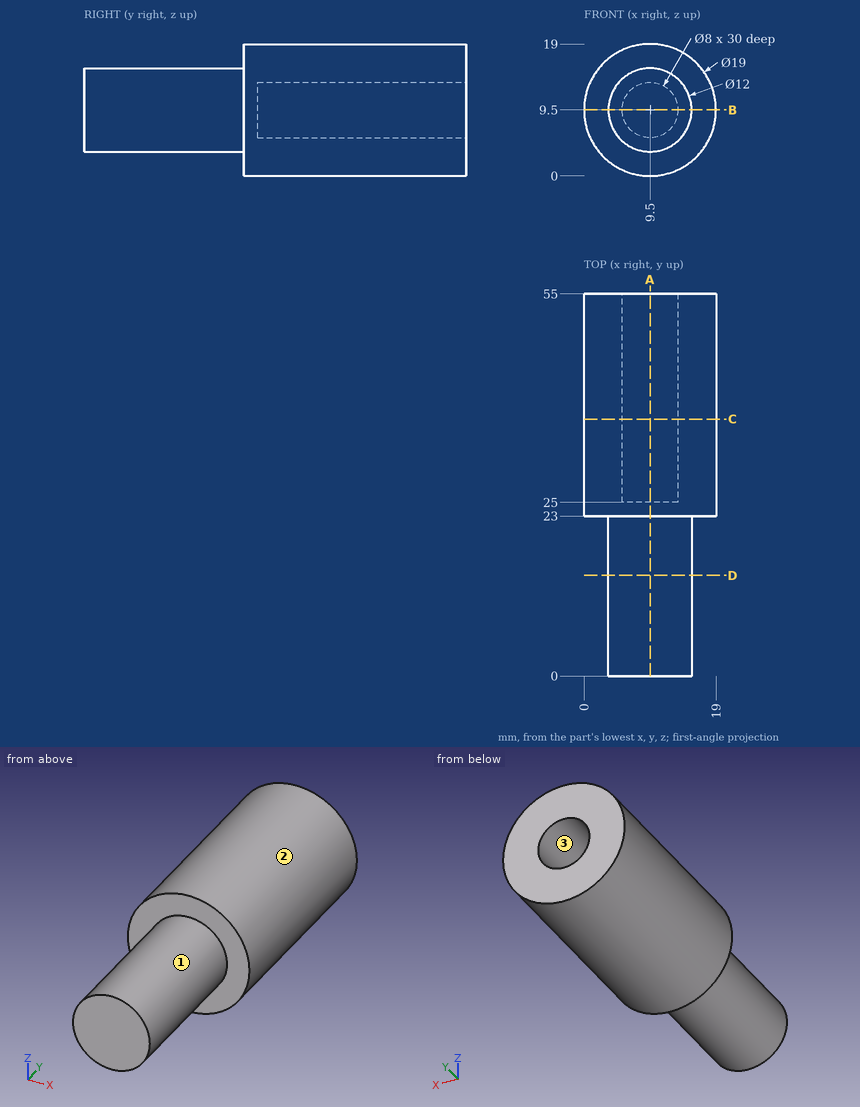
Could you check a few things on this drawing? It's one solid part, dimensions in mm from its lowest x, y, z. A direction names the side the tool comes from. Round coordinates to 2 decimals unless told otherwise and drop trailing zeros. Loops run counter-clockwise (first coordinate to the right, second up) from the corner with the lowest first, then second, coordinate; pieces in that order, holes last. Notation, with made-up numbers: M 43.5,28.5 L 79.5,28.5 A16 ccw 79.5,34.5 Z; hole C 40,35 d4. An arc over 180 degrees is marked long. Write each question's results on one line, items separated by ' | '. Start each with the question number.
(1) Will these pins go through, and if not, where does the flat tip stop? P1, Ø3, axis at y = 25.5, z = 4, coming from the -X side; P2, Ø5, axis at y = 35, z = 13.5, coming from the +X side; P3, Ø3, axis at y = 16, z = 3.5, coming from the -X side.
(2) On a 3-axis mill with a long thin cutter (end or side, diameter ignored), from which of +Z, -Z, +X, -X, +Y, -Y can I reach the whole of each face in a straight line? I mean the marked faces 1, 2 and 3. Say none if no direction works.
(3) I want a section at A-A (x = 9.5). Please give me the cut outline in (y, z), then the cut area to 3 significant figures.
(4) I want a section at D-D (y = 14.5). Please give me the cut outline in (x, z).
(5) I want a section at B-B (z = 9.5). Please give me the cut outline in (x, y), then the cut area to 3 significant figures.
(6) I want a section at C-C (y = 37). Please give me the cut outline in (x, z), then the cut area to 3 significant figures.
(7) If I drill on probe 1 along Z at (x, y) = (9.5, 44.25); probe 2 along Y at (x, z) = (17.5, 11.25); probe 3 along X at (y, z) = (31, 7), over which ranges is the centre line in solid material (lowest first)? Write a range as from..to.
Solved:
1) P1: stops at x = 0.88 | P2: stops at x = 18.88 | P3: stops at x = 5.53
2) face 1: -Y | face 2: +Y, -Y | face 3: +Y
3) outline: M 0,3.5 L 23,3.5 L 23,0 L 55,0 L 55,5.5 L 25,5.5 L 25,13.5 L 55,13.5 L 55,19 L 23,19 L 23,15.5 L 0,15.5 Z | area: 644 mm²
4) outline: C 9.5,9.5 d12
5) outline: M 0,23 L 3.5,23 L 3.5,0 L 15.5,0 L 15.5,23 L 19,23 L 19,55 L 13.5,55 L 13.5,25 L 5.5,25 L 5.5,55 L 0,55 Z | area: 644 mm²
6) outline: C 9.5,9.5 d19; hole C 9.5,9.5 d8 | area: 233 mm²
7) probe 1: z = 0..5.5, 13.5..19 | probe 2: y = 23..55 | probe 3: x = 0.33..6.38, 12.62..18.67
